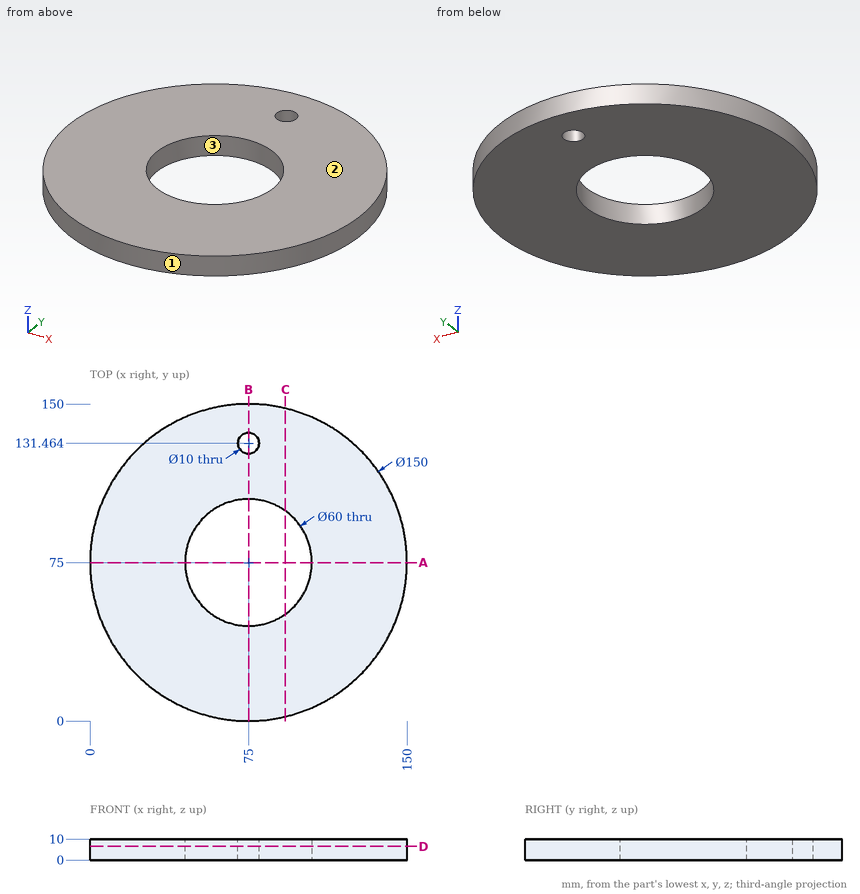
Geometry: see drawing. Coordinates: mm, zero at the bounding-box minimum. Coordinates: 2 decimals unless noted, no trailing zeros. Order: outer loops, then holes, each group sorted by start corner. A loop starts at its lowest first (then second) coordinate and runs counter-clockwise, first axis right, second up. Notation, with made-up numbers: M -37.5,5.25 L 11.5,5.25 A34 cw 11.5,42.25 Z; hole C -21.5,20 d9. An arc over 180 degrees is marked long. Answer in a Markdown table with one row per item. Add a question column.
Q1. Mould query, pull axis Y, two halves, no side actions, for the marked faces 1, 2 and 3. Classes: released by +Y, released by -Y, zero draft, split by the parting line, or undercut.
Q2. Section query B-B on x = 75. Return the cut outline in (y, z), and give its area (3 significant figures).
Q3. Contact query for flat-ended pins moving along their axis: P1, Ø3, axis at x = 66, z = 5.5, coming from the +Y side; P2, Ø1.5, axis at y = 86, z = 8.5, coming from the -X side; P3, Ø2, axis at x = 40.5, z = 9, coming from the +Y side. Output: stop coordinate, or through.
Q4. Section query C-C on x = 92.5. Return the cut outline in (y, z), and give its area (3 significant figures).
Q5. Section query D-D on z = 6.5. Return the cut outline in (x, y).
Q6. Section query A-A on y = 75. Return the cut outline in (x, z).
Q7. Line query: L1, parallel to Y at x = 75, z = 4; L2, parallel to Y at x = 74, z = 4 (1 decimal); L3, parallel to X at y = 131, z = 5. Output: solid intervals per line, ascending.
Completed:
| question | item | result |
|---|---|---|
| 1 | face 1 | split by the parting line |
| 1 | face 2 | zero draft |
| 1 | face 3 | undercut |
| 2 | outline | M 0,0 L 45,0 L 45,10 L 0,10 Z; M 105,0 L 126.46,0 L 126.46,10 L 105,10 Z; M 136.46,0 L 150,0 L 150,10 L 136.46,10 Z |
| 2 | area | 800 mm2 |
| 3 | P1 | stops at y = 149.62 |
| 3 | P2 | stops at x = 0.7 |
| 3 | P3 | stops at y = 142.1 |
| 4 | outline | M 2.07,0 L 50.63,0 L 50.63,10 L 2.07,10 Z; M 99.37,0 L 147.93,0 L 147.93,10 L 99.37,10 Z |
| 4 | area | 971 mm2 |
| 5 | outline | C 75,75 d150; hole C 75,75 d60; hole C 75,131.46 d10 |
| 6 | outline | M 0,0 L 45,0 L 45,10 L 0,10 Z; M 105,0 L 150,0 L 150,10 L 105,10 Z |
| 7 | L1 | y = 0 to 45, 105 to 126.46, 136.46 to 150 |
| 7 | L2 | y = 0 to 45, 105 to 126.6, 136.4 to 150 |
| 7 | L3 | x = 25.11 to 70.02, 79.98 to 124.89 |
